The listing builds one solid part. Answer for the finished solid, in the listing's coordinates (mm). A direction names the side the tool comes from. Coordinates: 2 decimals unless noted, no trailing zeros. Write each loop counter-clockwise with the first axis right and the second up, starting at its lowest first coordinate (ties: lowest second). Pieces come first, ordered by that corner, then holes. Notation, with made-up numbers: M 40.25,18.25 L 90.25,18.25 A16 ccw 90.25,32.25 Z; hole C 27.25,47 d10. An arc over 180 degrees is marked long. Answer as CSV lines item,"result".
```python
from build123d import *

# Parameters (mm, degrees)
SKETCH_1_W         = 75
SKETCH_1_H         = 162
BLOCKEXTRUDE_DEPTH = 70
FILLET_2_R         = 3
SHELL_START        = 3
SHELL_1_OUTLINE_W  = 159
SHELL_1_OUTLINE_H  = 64
SHELL_1_DEPTH      = 69
SKETCH_2_R         = 4.1
CABLE_ENTRY_DEPTH  = 192.752444574


# Read off the part's stored shape, not the designer's step: 抽壳1
with BuildPart() as part:
    # 草图1 → BlockExtrude (new body)
    with BuildSketch(Plane.XY):
        with Locations((37.5, 81)):
            Rectangle(SKETCH_1_W, SKETCH_1_H)
    extrude(amount=BLOCKEXTRUDE_DEPTH)

    # Fillet 2
    fillet_2_edges = [part.edges().sort_by_distance(p)[0] for p in [
        (75, 81, 70),
        (0, 81, 70),
        (75, 81, 0),
        (0, 81, 0),
    ]]
    fillet(fillet_2_edges, radius=FILLET_2_R)

    # 抽壳1 outline → 抽壳1 (cut)
    with BuildSketch(Plane.YZ.offset(SHELL_START)):
        with Locations((82.5, 35)):
            Rectangle(SHELL_1_OUTLINE_W, SHELL_1_OUTLINE_H)
    extrude(amount=SHELL_1_DEPTH, mode=Mode.SUBTRACT)

    # 草图2 → Cable_entry (cut, through all)
    with BuildSketch(Plane(origin=(0, 0, 0), x_dir=(-1, 0, 0), z_dir=(0, 0, -1))):
        with Locations((-37.5, 77)):
            Circle(SKETCH_2_R)
    extrude(amount=-CABLE_ENTRY_DEPTH, mode=Mode.SUBTRACT)


solid = part.part
```
Q1. A flat-ended cylindrical pin translates along its axis: pin 1 Ø5 at (x, z) = (56.5, 55.5) entering from +Y. Find the tip coordinate at first contact, or state that the pin passes through.
Output:
pin 1,"y = 3"
Q2. Straight lines are drawn through the part: line 1 (Z direction, x = 20, y = 111); line 2 (X direction, y = 113, z = 26); line 3 (Y direction, x = 37.5, z = 2.2). For each, find the intervals that lie inside material, in ascending order.
Output:
line 1,"0 to 3, 67 to 70"
line 2,"0 to 3, 72 to 75"
line 3,"0 to 72.9, 81.1 to 162"
Q3. For faces 1 (the cylindrical face through (38.034, 81.065, 68.479)), 2 (the flat face through (37, 81.4, 3)), determine the directions among +Z, -Z, +X, -X, +Y, -Y from which every point of the face is accessible in a straight line to the end or side of a thin tool.
Output:
face 1,"+Z, -Z"
face 2,"+Y"
Q4. Find section D-D (y = 142.5). Give the vertices of the cut face in (x, z).
Output:
outline,"M 0,3 A3 ccw 3,0 L 72,0 A3 ccw 75,3 L 75,67 A3 ccw 72,70 L 3,70 A3 ccw 0,67 Z; hole M 3,3 L 72,3 L 72,67 L 3,67 Z"
Q5. Find section A-A (x = 37.5). Give the vertices of the cut face in (y, z).
Output:
outline,"M 0,0 L 72.9,0 L 72.9,3 L 3,3 L 3,67 L 72.9,67 L 72.9,70 L 0,70 Z; M 81.1,0 L 162,0 L 162,3 L 81.1,3 Z; M 81.1,67 L 162,67 L 162,70 L 81.1,70 Z"
Q6. Find section C-C (z = 51.5). Give the vertices of the cut face in (x, y), and give its area (3 significant figures).
Output:
outline,"M 0,0 L 75,0 L 75,162 L 72,162 L 72,3 L 3,3 L 3,162 L 0,162 Z"
area,"1,180 mm2"
Q7. The mould has two halves that part along X. Classify faces 3 (the cylindrical face through (0.86, 82.13, 0.9)), 4 (the flat face through (37, 81.4, 67)), 5 (the cylindrical face through (74.14, 82.13, 0.9)): pulls with the +X half, pulls with the -X half, needs draft (parallel to the pull), parting line crosses it, or undercut.
Output:
face 3,"pulls with the -X half"
face 4,"undercut"
face 5,"pulls with the +X half"
Q8. Find section B-B (y = 77). Give the vertices of the cut face in (x, z).
Output:
outline,"M 0,3 A3 ccw 3,0 L 33.4,0 L 33.4,3 L 3,3 L 3,67 L 33.4,67 L 33.4,70 L 3,70 A3 ccw 0,67 Z; M 41.6,0 L 72,0 A3 ccw 75,3 L 75,67 A3 ccw 72,70 L 41.6,70 L 41.6,67 L 72,67 L 72,3 L 41.6,3 Z"
